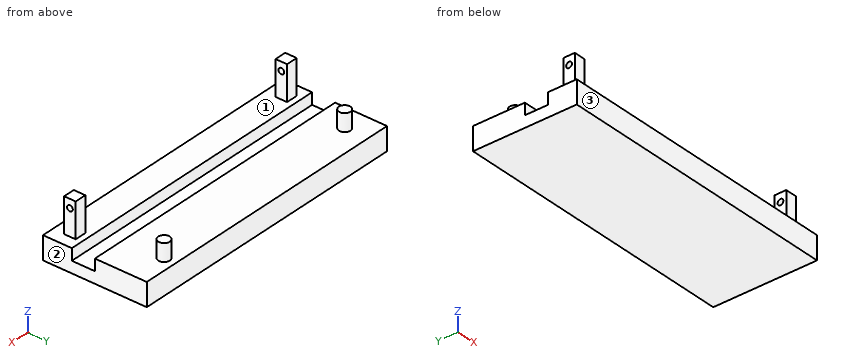
```python
from build123d import *

# Parameters (mm, degrees)
F0_W      = 250
F0_H      = 90
F1_DEPTH  = 20
F2_R      = 5
F3_DEPTH  = 15
F4_W      = 250
F4_H      = 20
F5_DEPTH  = 10
F6_W      = 10
F6_H      = 10
F7_DEPTH  = 30
F8_R      = 2.5
F9_DEPTH  = 20.001
F10_R     = 2.5
F11_DEPTH = 20.001


with BuildPart() as f1:
    # F0 (on Top) → F1 (new body)
    with BuildSketch(Plane.XY):
        Rectangle(F0_W, F0_H)
    extrude(amount=F1_DEPTH)

    # F2 (on face) → F3 (join)
    with BuildSketch(Plane.XY.offset(20)):
        with Locations((95, 35)):
            Circle(F2_R)
        with Locations((-105, 25)):
            Circle(F2_R)
    extrude(amount=F3_DEPTH)

    # F4 (on face) → F5 (cut)
    with BuildSketch(Plane.XY.offset(20)):
        with Locations((0, -10)):
            Rectangle(F4_W, F4_H)
    extrude(amount=-F5_DEPTH, mode=Mode.SUBTRACT)

    # F6 (on face) → F7 (join)
    with BuildSketch(Plane.XY.offset(20)):
        with Locations((-110, -30)):
            Rectangle(F6_W, F6_H)
        with Locations((110, -30)):
            Rectangle(F6_W, F6_H)
    extrude(amount=F7_DEPTH)

    # F8 (on face) → F9 (cut, through all)
    with BuildSketch(Plane.YZ.offset(-105)):
        with Locations((-30, 42.5)):
            Circle(F8_R)
    extrude(amount=-F9_DEPTH, mode=Mode.SUBTRACT)

    # F10 (on face) → F11 (cut, through all)
    with BuildSketch(Plane(origin=(105, 0, 0), x_dir=(0, -1, 0), z_dir=(-1, 0, 0))):
        with Locations((30, 42.5)):
            Circle(F10_R)
    extrude(amount=-F11_DEPTH, mode=Mode.SUBTRACT)


solid = f1.part
```
Geometry check sheet. Reference: the model listing, model coordinates, mm. Face numbers are marked on the shaded views. Coordinates: 2 decimals unless noted, no trailing zeros. Loops run counter-clockwise (first coordinate to the right, second up) from the corner with the lowest first, then second, coordinate; pieces in that order, holes last.
Item 1: Sectioned sample at C-C, the plane x = -36.5. Record the boundary of the cut face in (y, z), then the cut area to 3 significant figures.
Item 2: Thickness scan on line 1 (Z direction, x = 112, y = -30); line 2 (Y direction, x = 33, z = 17.5); line 3 (Y direction, x = -108, z = 42). Record the ranges inside material, lowest first.
Item 3: Go/stop test with flat-tipped pins: pin 1 Ø4 at (x, y) = (77.5, -20.5) entering from +Z; pin 2 Ø11 at (x, z) = (109, 39.5) entering from -Y; pin 3 Ø3 at (y, z) = (-32, 29.5) entering from +X. Record where each tip stops, or that it passes through.
Item 4: Sectioned sample at D-D, the plane z = 15. Record the boundary of the cut face in (x, y).
Item 5: Sectioned sample at B-B, the plane z = 42.5. Record the boundary of the cut face in (x, y).
Item 6: Sectioned sample at A-A, the plane y = -30. Record the boundary of the cut face in (x, z), then the cut area to 3 significant figures.
Item 7: Release check for a two-part mould opening along X. For the marked faces 1, 2 and 3 record: released by +X, released by -X, zero draft, split by the parting line, or undercut.
Check result:
1. outline: (-45, 0) - (45, 0) - (45, 20) - (0, 20) - (0, 10) - (-20, 10) - (-20, 20) - (-45, 20) - close
1. area: 1,600 mm2
2. line 1: z = 0 to 40, 45 to 50
2. line 2: y = -45 to -20, 0 to 45
2. line 3: y = -35 to -32.45, -27.55 to -25
3. pin 1: stops at z = 20
3. pin 2: stops at y = -35
3. pin 3: stops at x = 115
4. outline: (-125, -45) - (125, -45) - (125, -20) - (-125, -20) - close; (-125, 0) - (125, 0) - (125, 45) - (-125, 45) - close
5. outline: (-115, -35) - (-105, -35) - (-105, -32.5) - (-115, -32.5) - close; (-115, -27.5) - (-105, -27.5) - (-105, -25) - (-115, -25) - close; (105, -35) - (115, -35) - (115, -32.5) - (105, -32.5) - close; (105, -27.5) - (115, -27.5) - (115, -25) - (105, -25) - close
6. outline: (-125, 0) - (125, 0) - (125, 20) - (115, 20) - (115, 40) - (105, 40) - (105, 20) - (-105, 20) - (-105, 40) - (-115, 40) - (-115, 20) - (-125, 20) - close; (-115, 45) - (-105, 45) - (-105, 50) - (-115, 50) - close; (105, 45) - (115, 45) - (115, 50) - (105, 50) - close
6. area: 5,500 mm2
7. face 1: undercut
7. face 2: released by +X
7. face 3: zero draft
